Could you check a few things on this model? Use its own coordinates, in mm. Face numbers are marked on the shaded views. A direction names the side the tool comes from. Give positions to 0.01 mm unless a question says otherwise; leave off trailing zeros. Loops run counter-clockwise (first coordinate to the right, second up) from the corner with the lowest first, then second, coordinate; pieces in that order, holes last. Notation, with made-up numbers: (-5.75, 60.25) - (51.25, 60.25) arc R30 ccw to (51.25, 92.25) - close; hole circle Ø10 at (33, 76). An arc over 180 degrees is marked (long way). Write each question's results on one line, items separated by ' | '. Start each with the question number.
(1) Suppose I cut it at A-A (y = 0). Please give me the cut outline in (x, z).
(2) I need wall thicknesses on line 1 (Y direction, x = 49.3, z = 0); line 2 (Z direction, x = -37.5, y = -0.75); line 3 (X direction, y = -6.25, z = 20.5). Which ranges of each line are inside material? Lowest first, please.
(3) For pin 1 (5 mm diameter, centred on y = -1.5, z = 21, fed in from -X); pin 2 (3 mm diameter, centred on x = -2.5, y = -5.5, fed in from +Z); pin 3 (8 mm diameter, centred on y = -6, z = 19, fed in from -X), each with a flat end and sliding along its axis, tell me the tip position at first contact or that it passes through.
(4) Suppose I cut it at C-C (z = 31). Please give me the cut outline in (x, y), and give its area (3 significant figures).
(5) Suppose I cut it at D-D (z = 0). Please give me the cut outline in (x, y).
(6) On a 3-axis mill with a long thin cutter (end or side, diameter ignored), from which of +Z, -Z, +X, -X, +Y, -Y can I reach the whole of each face in a straight line? I mean the marked faces 1 and 2. Say none if no direction works.
(7) Suppose I cut it at B-B (x = 0). Please give me the cut outline in (y, z).
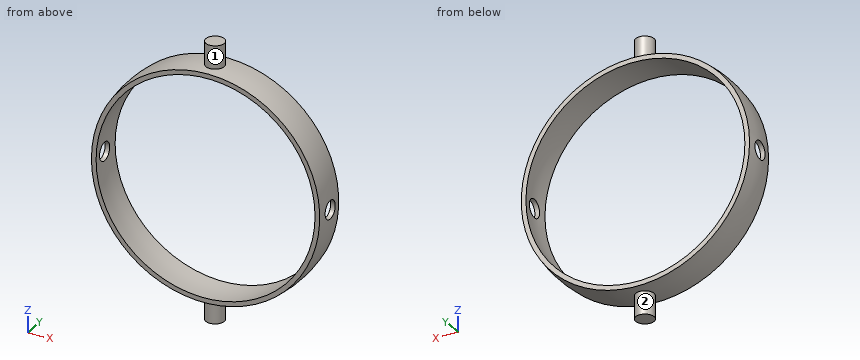
from build123d import *

# Parameters (mm, degrees)
SKETCH2_R               = 4
CUT_EXTRUDE1_DEPTH      = 51
CUT_EXTRUDE1_DEPTH_BACK = 51
SKETCH6_R               = 4
BOSS_EXTRUDE1_DEPTH     = 10.160257


with BuildPart() as part:
    # Sketch1 → Revolve1 (revolve)
    with BuildSketch(Plane.XY):
        with BuildLine():
            Line((-49.434299833, 7.5), (-47.410441888, 7.5))
            ThreePointArc((-47.410441888, 7.5), (-48, 0), (-47.410441888, -7.5))
            Line((-47.410441888, -7.5), (-49.434299833, -7.5))
            ThreePointArc((-49.434299833, -7.5), (-50, 0), (-49.434299833, 7.5))
        make_face()
    revolve(axis=Axis((0, 31.203935911, 0), (0, -1, 0)))

    # Sketch2 → Cut-Extrude1 (cut, two sides)
    with BuildSketch(Plane(origin=(0, 0, 0), x_dir=(0, 0, -1), z_dir=(1, 0, 0))) as cut_extrude1_sk:
        Circle(SKETCH2_R)
    extrude(amount=CUT_EXTRUDE1_DEPTH, mode=Mode.SUBTRACT)
    extrude(cut_extrude1_sk.sketch, amount=-CUT_EXTRUDE1_DEPTH_BACK, mode=Mode.SUBTRACT)

    # Sketch6 → Boss-Extrude1 (add)
    with BuildSketch(Plane.XY.offset(60)):
        Circle(SKETCH6_R)
    boss_extrude1 = extrude(amount=-BOSS_EXTRUDE1_DEPTH)

    # Mirror1: Boss-Extrude1 across plane
    add(boss_extrude1.mirror(Plane.XY))

    # Sketch8 → Cut-Revolve1 (revolve, cut)
    with BuildSketch(Plane(origin=(0, 0, 0), x_dir=(0, 0, -1), z_dir=(1, 0, 0))):
        with BuildLine():
            Line((0, 70), (0, 60))
            ThreePointArc((0, 60), (-60, 0), (0, -60))
            Line((0, -60), (0, -70))
            ThreePointArc((0, -70), (-70, 0), (0, 70))
        make_face()
    revolve(axis=Axis((0, 45.192031549, 0), (0, -1, 0)), mode=Mode.SUBTRACT)


solid = part.part
Output values:
1) outline: (-49.84, -4) arc R50 ccw to (-4, -49.84) - (-4, -59.87) arc R60 ccw to (4, -59.87) - (4, -49.84) arc R50 ccw to (49.84, -4) - (47.83, -4) arc R48 cw to (-47.83, -4) - close; (-49.84, 4) - (-47.83, 4) arc R48 cw to (47.83, 4) - (49.84, 4) arc R50 ccw to (4, 49.84) - (4, 59.87) arc R60 ccw to (-4, 59.87) - (-4, 49.84) arc R50 ccw to start
2) line 1: -7.5 to -4, 4 to 7.5 | line 2: -33.06 to -29.95, 29.95 to 33.06 | line 3: -45.17 to -42.95, 42.95 to 45.17
3) pin 1: x = -46.43 | pin 2: z = 49.79 | pin 3: x = -47.4
4) outline: (-38.51, -7.5) - (-35.87, -7.5) arc R36.65 cw to (-35.87, 7.5) - (-38.51, 7.5) arc R39.23 ccw to start; (35.87, -7.5) - (38.51, -7.5) arc R39.23 ccw to (38.51, 7.5) - (35.87, 7.5) arc R36.65 cw to start | area: 78.0 mm2
5) outline: (-49.84, -4) arc R50 ccw to (-49.43, -7.5) - (-47.41, -7.5) arc R48 cw to (-47.83, -4) - close; (-49.84, 4) - (-47.83, 4) arc R48 cw to (-47.41, 7.5) - (-49.43, 7.5) arc R50 ccw to start; (47.41, -7.5) - (49.43, -7.5) arc R50 ccw to (49.84, -4) - (47.83, -4) arc R48 cw to start; (47.41, 7.5) arc R48 cw to (47.83, 4) - (49.84, 4) arc R50 ccw to (49.43, 7.5) - close
6) face 1: +Z | face 2: -Z
7) outline: (-7.5, -49.43) arc R50 ccw to (-4, -49.84) - (-4, -59.87) arc R60 ccw to (4, -59.87) - (4, -49.84) arc R50 ccw to (7.5, -49.43) - (7.5, -47.41) arc R48 cw to (-7.5, -47.41) - close; (-7.5, 47.41) arc R48 cw to (7.5, 47.41) - (7.5, 49.43) arc R50 ccw to (4, 49.84) - (4, 59.87) arc R60 ccw to (-4, 59.87) - (-4, 49.84) arc R50 ccw to (-7.5, 49.43) - close
